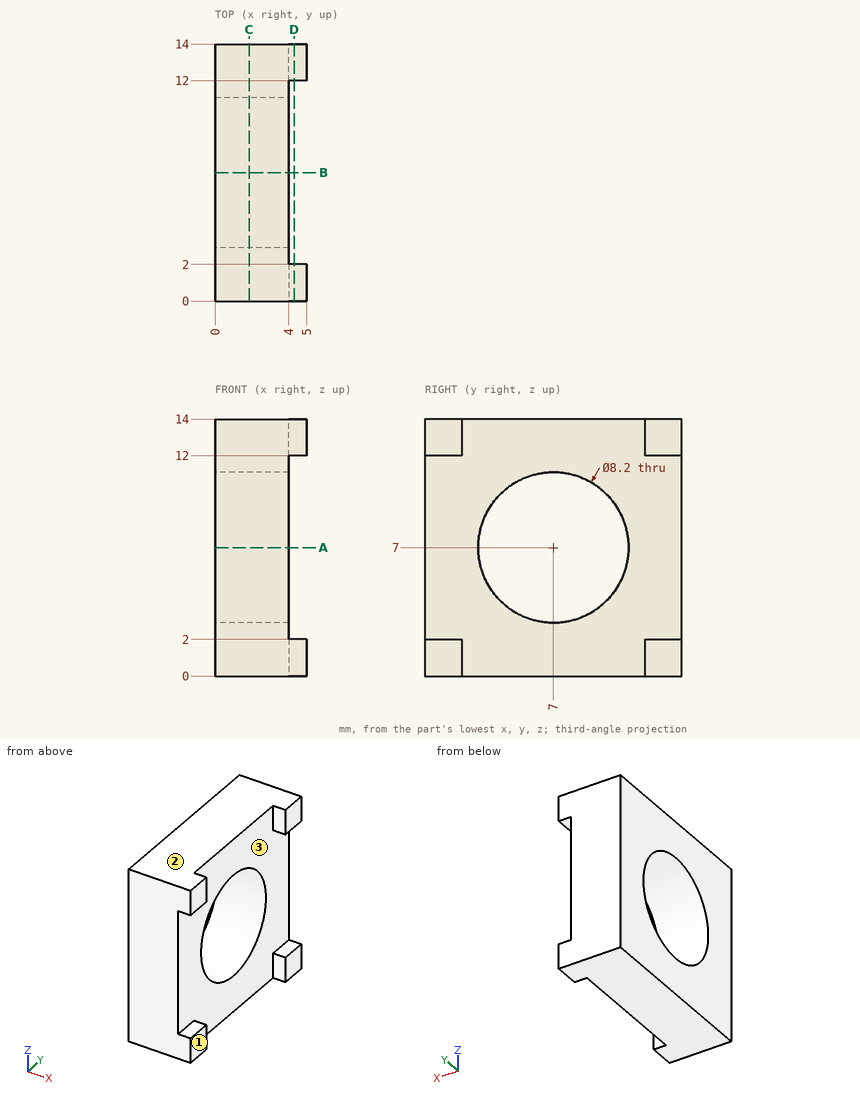
Input: dimensioned drawing with shaded views. Units: mm. Origin: part minimum x, y, z. Coordinates: 2 decimals unless noted, no trailing zeros. Order: outer loops, then holes, each group sorted by start corner. A loop starts at its lowest first (then second) coordinate and runs counter-clockwise, first axis right, second up. Notation, with made-up numbers: (38, 33.5) - (52, 33.5) arc R24 ccw to (52, 70.5) - close; hole circle Ø10 at (-38.5, 70.25). An arc over 180 degrees is marked (long way). Put each result on its own line as item: value.
1. Contact query for flat-ended pins moving along their axis: pin 1 Ø1.1 at (x, y) = (4.5, 13.5) entering from -Z; pin 2 Ø2 at (y, z) = (9.5, 2.5) entering from +X; pin 3 Ø1 at (y, z) = (4.5, 9) entering from -X. Output: stop coordinate, or through.
Report:
pin 1: stops at z = 0
pin 2: stops at x = 4
pin 3: passes through
2. Cut plane C-C on x = 1.85. Return the cut outline in (y, z), then the cut area to 3 significant figures.
Report:
outline: (0, 0) - (14, 0) - (14, 14) - (0, 14) - close; hole circle Ø8.2 at (7, 7)
area: 143 mm2
3. Cut plane A-A on z = 7. Return the cut outline in (x, y).
Report:
outline: (0, 0) - (4, 0) - (4, 2.9) - (0, 2.9) - close; (0, 11.1) - (4, 11.1) - (4, 14) - (0, 14) - close
4. Draft query along Z for the marked faces 1, 2 and 3. Return one class per face: pulls with the +Z half, pulls with the -Z half, needs draft (parallel to the pull), parting line crosses it, or undercut.
Report:
face 1: needs draft
face 2: pulls with the +Z half
face 3: undercut
5. Line query: line 1 along Y through (x, z) = (4.7, 12.25); line 2 along Z through (x, y) = (2.4, 7); line 3 along X through (y, z) = (4.5, 11). Output: solid intervals per line, ascending.
Report:
line 1: y = 0 to 2, 12 to 14
line 2: z = 0 to 2.9, 11.1 to 14
line 3: x = 0 to 4
6. Cut plane D-D on x = 4.3. Return the cut outline in (y, z).
Report:
outline: (0, 0) - (2, 0) - (2, 2) - (0, 2) - close; (0, 12) - (2, 12) - (2, 14) - (0, 14) - close; (12, 0) - (14, 0) - (14, 2) - (12, 2) - close; (12, 12) - (14, 12) - (14, 14) - (12, 14) - close
